Geometry: final body of the model. Coordinates: model frame, mm. A direction names the side the tool comes from. Give positions to 0.01 mm unless a question says otherwise; leave off trailing zeros. Order: outer loops, then holes, each group sorted by start corner. A loop starts at its lowest first (then second) coordinate and runs counter-clockwise, first axis right, second up. Notation, with made-up numbers: (19, -20.75) - (30, -20.75) arc R22 cw to (30, 5.25) - close; hole circle Ø11 at (34.25, 57.25). An arc over 180 degrees is marked (long way). One line per question, with ' | ' between items. Start each with the question number.
Autodesk Inventor part; units mm, degrees
ref_plane "YZ Plane" through (0, 0, 0) normal (1, 0, 0) x (0, 1, 0)
ref_plane "XZ Plane" through (0, 0, 0) normal (0, 1, 0) x (-1, 0, 0)
ref_plane "XY Plane" through (0, 0, 0) normal (0, 0, 1) x (1, 0, 0)
sketch "Sketch1" plane through (0, 0, 0) normal (0, 0, 1) x (1, 0, 0)
  circle A0 centre (-414.4261, -56.251) radius 4.7625
  point P0 (0, 0)
  dimension "d0" = 9.525
extrude "Extrusion1" add sketch "Sketch1" against normal blind 19.05
sketch "Sketch2" plane through (-414.4261, -56.251, 0) normal (0, 0, 1) x (1, 0, 0)
  circle A0 centre (0, 0) radius 4.7625
  line L0 (-8.2489, 0) -> (-4.1244, 7.1437)
  line L1 (-4.1244, 7.1437) -> (4.1244, 7.1438)
  line L2 (4.1244, 7.1438) -> (8.2489, 0)
  line L3 (8.2489, 0) -> (4.1244, -7.1437)
  line L4 (4.1244, -7.1437) -> (-4.1244, -7.1438)
  line L5 (-4.1244, -7.1438) -> (-8.2489, 0)
  point P0 (414.4261, 56.251)
  dimension "d3" = 14.2875
extrude "Extrusion2" add sketch "Sketch2" along normal blind 3.175 contours A0 | L0 L1 L2 L3 L4 L5
thread "Thread1"
chamfer "Chamfer1" distance 0.508 angle 45 1 edges at (-419.1886, -56.251, -19.05)
properties part number "375 bolt x4" material "Steel"
(1) Access query for faces 1 (the flat face through (-420.584, -59.873, 1.565)), 2 (the cylindrical face through (-419.184, -56.042, -9.141)). Directions: +Z, -Z, +X, -X, +Y, -Y. A direction counts if a zero-diameter tool reaches every point of the face in a straight line with its end or side. Return the directions, or none.
(2) Cut plane A-A, the plane z = -9. Return the cut outline in (x, y) (1 decimal), plus the area to 3 significant figures.
(3) Cut plane C-C, the plane y = -62.25. Return the cut outline in (x, z) (3 decimals), plus the area to 3 significant figures.
(4) Material intervals for line 1 along X through (y, z) = (-56, -1); line 2 along Z through (x, y) = (-407.25, -56.25) (3 decimals); line 3 along Y through (x, z) = (-414.25, -15), sorted ascending. Write a range as from..to.
(5) Contact query for flat-ended pins moving along their axis: P1, Ø5, axis at y = -61, z = -16.5, coming from the -X side; P2, Ø4, axis at x = -419.5, z = -12, coming from the -Y side; P3, Ø5, axis at x = -408.5, z = -3.5, coming from the +Y side. Output: stop coordinate, or through.
(6) Cut plane B-B, the plane x = -408.5. Return the cut outline in (y, z) (3 decimals).
Results are:
1) face 1: +Z, -Z, -X, -Y | face 2: -Z
2) outline: circle Ø9.5 at (-414.4, -56.3) | area: 71.3 mm2
3) outline: (-419.211, 0) - (-409.641, 0) - (-409.641, 3.175) - (-419.211, 3.175) - close | area: 30.4 mm2
4) line 1: -419.18..-409.67 | line 2: 0..3.175 | line 3: -61.01..-51.49
5) P1: x = -418.62 | P2: y = -59.89 | P3: y = -52.94
6) outline: (-60.274, 0) - (-52.228, 0) - (-52.228, 3.175) - (-60.274, 3.175) - close
